Work out the finished part from the listing and answer in its coordinate system (mm). Face numbers are marked on the shaded views. A direction names the side the tool comes from. Coordinates: 2 decimals unless noted, no trailing zeros. Order: outer loops, then holes, each group sorted by start corner. A loop starts at its lowest first (then second) coordinate and runs counter-clockwise, first axis right, second up. Notation, with made-up numbers: M 7.5,-13 L 54.5,-13 A32 ccw 54.5,25 Z; hole C 70.5,52.25 d9. An arc over 180 degrees is marked long. Use a Markdown table: item, result.
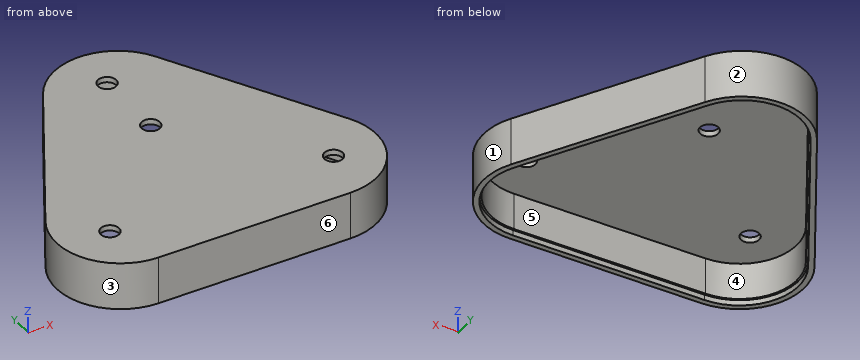
from build123d import *

# Parameters (mm, degrees)
RESSALTO_EXTRUS_O1_DEPTH = 3
RESSALTO_EXTRUS_O2_DEPTH = 20
RESSALTO_EXTRUS_O3_DEPTH = 3
ESBO_O4_R                = 5
CORTE_EXTRUS_O1_DEPTH    = 3


with BuildPart() as part:
    # Esboço1 → Ressalto-extrusão1 (new body)
    with BuildSketch(Plane.XY):
        with BuildLine():
            Line((51.961524227, -65), (-51.961524227, -65))
            ThreePointArc((-51.961524227, -65), (-82.27241336, -47.5), (-82.27241336, -12.5))
            Line((-82.27241336, -12.5), (-30.310889132, 77.5))
            ThreePointArc((-30.310889132, 77.5), (0, 95), (30.310889132, 77.5))
            Line((30.310889132, 77.5), (82.27241336, -12.5))
            ThreePointArc((82.27241336, -12.5), (82.27241336, -47.5), (51.961524227, -65))
        make_face()
        with BuildLine():
            Line((51.961524227, -62), (-51.961524227, -62))
            ThreePointArc((-51.961524227, -62), (-79.674337148, -46), (-79.674337148, -14))
            Line((-79.674337148, -14), (-27.712812921, 76))
            ThreePointArc((-27.712812921, 76), (0, 92), (27.712812921, 76))
            Line((27.712812921, 76), (79.674337148, -14))
            ThreePointArc((79.674337148, -14), (79.674337148, -46), (51.961524227, -62))
        make_face(mode=Mode.SUBTRACT)
    extrude(amount=RESSALTO_EXTRUS_O1_DEPTH)

    # Esboço2 → Ressalto-extrusão2 (add)
    with BuildSketch(Plane.XY.offset(3)):
        with BuildLine():
            Line((-51.961524227, -65), (51.961524227, -65))
            ThreePointArc((51.961524227, -65), (82.27241336, -47.5), (82.27241336, -12.5))
            Line((82.27241336, -12.5), (30.310889132, 77.5))
            ThreePointArc((30.310889132, 77.5), (0, 95), (-30.310889132, 77.5))
            Line((-30.310889132, 77.5), (-82.27241336, -12.5))
            ThreePointArc((-82.27241336, -12.5), (-82.27241336, -47.5), (-51.961524227, -65))
        make_face()
        with BuildLine():
            Line((-51.961524227, -61), (51.961524227, -61))
            ThreePointArc((51.961524227, -61), (78.808311744, -45.5), (78.808311744, -14.5))
            Line((78.808311744, -14.5), (26.846787517, 75.5))
            ThreePointArc((26.846787517, 75.5), (0, 91), (-26.846787517, 75.5))
            Line((-26.846787517, 75.5), (-78.808311744, -14.5))
            ThreePointArc((-78.808311744, -14.5), (-78.808311744, -45.5), (-51.961524227, -61))
        make_face(mode=Mode.SUBTRACT)
    extrude(amount=RESSALTO_EXTRUS_O2_DEPTH)

    # Esboço3 → Ressalto-extrusão3 (add)
    with BuildSketch(Plane.XY.offset(23)):
        with BuildLine():
            Line((-30.310889132, 77.5), (-82.27241336, -12.5))
            ThreePointArc((-82.27241336, -12.5), (-82.27241336, -47.5), (-51.961524227, -65))
            Line((-51.961524227, -65), (51.961524227, -65))
            ThreePointArc((51.961524227, -65), (82.27241336, -47.5), (82.27241336, -12.5))
            Line((82.27241336, -12.5), (30.310889132, 77.5))
            ThreePointArc((30.310889132, 77.5), (0, 95), (-30.310889132, 77.5))
        make_face()
    extrude(amount=RESSALTO_EXTRUS_O3_DEPTH)

    # Esboço4 → Corte-extrusão1 (cut)
    with BuildSketch(Plane.XY.offset(26)):
        with Locations((0, 70)):
            Circle(ESBO_O4_R)
        with Locations((60.621778265, -35)):
            Circle(ESBO_O4_R)
        with Locations((-60.621778265, -35)):
            Circle(ESBO_O4_R)
        with Locations((0, 30)):
            Circle(ESBO_O4_R)
    extrude(amount=-CORTE_EXTRUS_O1_DEPTH, mode=Mode.SUBTRACT)


solid = part.part
1. For a pull along X with two mould halves and no side action, classify the marked faces 1, 2, 3 and 4 as +X half, -X half, draft (parallel to the pull), parting line (faces both ways), or undercut.
Answers below:
| item | result |
|---|---|
| face 1 | +X half |
| face 2 | parting line |
| face 3 | -X half |
| face 4 | undercut |
2. Section A-A on x = 0 is taken. Determine the outline of the cut face in (y, z), then the cut area to 3 significant figures.
Answers below:
| item | result |
|---|---|
| outline | M -65,0 L -62,0 L -62,3 L -61,3 L -61,23 L 25,23 L 25,26 L -65,26 Z; M 35,23 L 65,23 L 65,26 L 35,26 Z; M 75,23 L 91,23 L 91,3 L 92,3 L 92,0 L 95,0 L 95,26 L 75,26 Z |
| area | 598 mm² |
3. Find the intervals of material crossed by probe 1 along Y at (x, z) = (0, 24.2); probe 2 along Z at (x, y) = (-48, -32); probe 3 along X at (y, z) = (-35, 13), in increasing order.
Answers below:
| item | result |
|---|---|
| probe 1 | -65 to 25, 35 to 65, 75 to 95 |
| probe 2 | 23 to 26 |
| probe 3 | -86.6 to -82.56, 82.56 to 86.6 |
4. Section D-D on y = -35 is taken. Determine the outline of the cut face in (x, z).
Answers below:
| item | result |
|---|---|
| outline | M -86.6,0 L -83.57,0 L -83.57,3 L -82.56,3 L -82.56,23 L -65.62,23 L -65.62,26 L -86.6,26 Z; M -55.62,23 L 55.62,23 L 55.62,26 L -55.62,26 Z; M 65.62,23 L 82.56,23 L 82.56,3 L 83.57,3 L 83.57,0 L 86.6,0 L 86.6,26 L 65.62,26 Z |
5. Flat-ended cylindrical pins translate along their axes: P1, Ø5, axis at x = 56.5, z = 19.5, coming from the -Y side; P2, Ø0.9, axis at x = -11.5, z = 1, coming from the +Y side; P3, Ø3, axis at y = -9.5, z = 4, coming from the +X side; P4, Ø16, axis at x = -60.62, y = -35, coming from the +Z side. Find the tip coordinate at first contact, or state that the pin passes through.
Answers below:
| item | result |
|---|---|
| P1 | y = -64.94 |
| P2 | y = 93.21 |
| P3 | x = 81.41 |
| P4 | z = 26 |
6. Section B-B on y = 30 is taken. Determine the outline of the cut face in (x, z), then the cut area to 3 significant figures.
Answers below:
| item | result |
|---|---|
| outline | M -57.74,0 L -54.27,0 L -54.27,3 L -53.12,3 L -53.12,23 L -5,23 L -5,26 L -57.74,26 Z; M 5,23 L 53.12,23 L 53.12,3 L 54.27,3 L 54.27,0 L 57.74,0 L 57.74,26 L 5,26 Z |
| area | 522 mm² |
7. Section C-C on z = 19 is taken. Determine the outline of the cut face in (x, y).
Answers below:
| item | result |
|---|---|
| outline | M -82.27,-12.5 A35 ccw -51.96,-65 L 51.96,-65 A35 ccw 82.27,-12.5 L 30.31,77.5 A35 ccw -30.31,77.5 Z; hole M -78.81,-14.5 A31 ccw -51.96,-61 L 51.96,-61 A31 ccw 78.81,-14.5 L 26.85,75.5 A31 ccw -26.85,75.5 Z |
8. For the marked faces 5 and 6, determine the directions among +Z, -Z, +X, -X, +Y, -Y from which every point of the face is accessible in a straight line to the end or side of a thin tool.
Answers below:
| item | result |
|---|---|
| face 5 | -Z |
| face 6 | +Z, -Z, +X, -X, -Y |
